Check sheet for the modelled part. Datum: model origin and axes. Units: mm. Face numbers are marked on the shaded views. A direction names the side the tool comes from. Round coordinates to 2 decimals unless told otherwise and drop trailing zeros. Order: outer loops, then holes, each group sorted by start corner. A loop starts at its lowest first (then second) coordinate and runs counter-clockwise, first axis right, second up. Notation, with made-up numbers: (89, 50.25) -> (99, 50.25) arc R21 ccw to (99, 89.25) -> close; hole circle Ø10 at (15.5, 84). An arc over 180 degrees is marked (long way). Answer in a Markdown table with one row per item. Add a question column.
1. Sectioned sample at B-B, the plane y = -103.5. Record the boundary of the cut face in (x, z).
2. Draft check along X on the marked faces 4, 5 and 6. Enter one of: +X half, -X half, draft (parallel to the pull), parting line (faces both ways), or undercut.
3. Material ranges on L1, parallel to Y at x = -21, z = -54; L2, parallel to X at y = -60.5, z = -39; L3, parallel to X at y = -79, z = -50, recorded low to high. Write a range as from..to.
4. Depth check by flat-ended pin: P1, Ø6, axis at y = -40.5, z = 13, coming from the +X side; P2, Ø8, axis at x = -46.5, z = -39, coming from the -Y side; P3, Ø8.5, axis at x = -23, y = -77, coming from the -Z side. Enter the tip coordinate at first touch or a pass-through.
5. Sectioned sample at D-D, the plane x = -25. Record the boundary of the cut face in (y, z), then the cut area to 3 significant figures.
6. Access from +Z, -Z, +X, -X, +Y, -Y to the whole of each face (thin tool, end or side, straight path). Record for the marked faces 1, 2 and 3.
7. Sectioned sample at A-A, the plane x = 4.5. Record the boundary of the cut face in (y, z), then the cut area to 3 significant figures.
8. Sectioned sample at C-C, the plane z = -14.5. Count the separate pieces of the cut face and the enclosed holes in it, then the cut area to 3 significant figures.
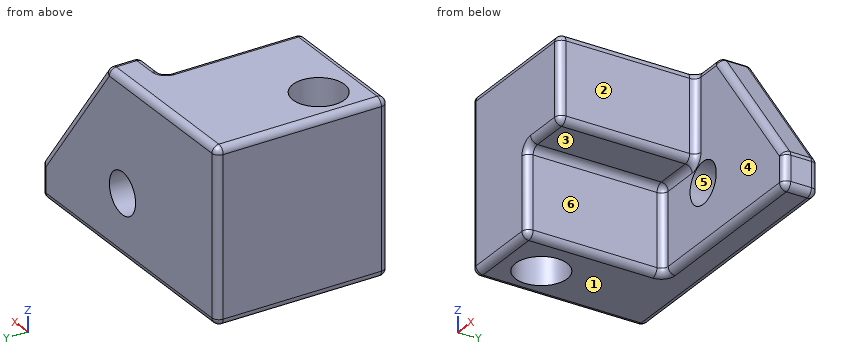
```python
from build123d import *

# Parameters (mm, degrees)
F0_W     = 203.2
F0_H     = 127
F1_DEPTH = 127
F3_DEPTH = 101.6
F4_SIZE2 = 101.6
F4_SIZE  = 76.2
F5_R     = 5.08
F6_R     = 15.24
F7_DEPTH = 25.4
F8_R     = 19.05
F9_DEPTH = 127


with BuildPart() as f1:
    # F0 (on Front) → F1 (new body)
    with BuildSketch(Plane.XZ):
        with Locations((-8.4275533497, -0.4033995528)):
            Rectangle(F0_W, F0_H)
    extrude(amount=F1_DEPTH)

    # F2 (on face) → F3 (cut)
    with BuildSketch(Plane.XZ.offset(127)):
        Polygon((-46.5275533497, -0.4033995528), (-46.5275533497, -63.9033995528), (93.1724466503, -63.9033995528), (93.1724466503, 63.0966004472), (-8.4275533497, 63.0966004472), (-8.4275533497, -0.4033995528), align=None)
    extrude(amount=-F3_DEPTH, mode=Mode.SUBTRACT)

    # F4
    f4_edges = [f1.edges().sort_by_distance(p)[0] for p in [
        (93.172447, -12.7, 63.0966),
    ]]
    f4_side = f1.faces().sort_by_distance((-42.29422, -55.033333, 63.0966))[0]
    chamfer(f4_edges, length=F4_SIZE, length2=F4_SIZE2, reference=f4_side)

    # F5
    f5_edges = [f1.edges().sort_by_distance(p)[0] for p in [
        (-46.527553, 0, 63.0966),
        (16.972447, -12.7, 63.0966),
        (-110.027553, -63.5, 63.0966),
        (4.272447, -25.4, 63.0966),
        (-59.227553, -127, 63.0966),
        (-8.427553, -76.2, 63.0966),
        (-8.427553, -127, 31.3466),
        (-27.477553, -127, -0.4034),
        (-46.527553, -127, -32.1534),
        (-78.277553, -127, -63.9034),
        (-110.027553, -127, -0.4034),
        (-8.427553, -76.2, -0.4034),
        (-8.427553, -25.4, 31.3466),
        (-46.527553, -76.2, -0.4034),
        (-46.527553, -76.2, -63.9034),
        (-46.527553, -25.4, -32.1534),
        (93.172447, -25.4, -51.2034),
        (55.072447, -25.4, 12.2966),
        (23.322447, -25.4, -63.9034),
        (-27.477553, -25.4, -0.4034),
        (55.072447, 0, 12.2966),
        (93.172447, -12.7, -38.5034),
        (93.172447, 0, -51.2034),
        (93.172447, -12.7, -63.9034),
        (-110.027553, -63.5, -63.9034),
        (-110.027553, 0, -0.4034),
        (-8.427553, 0, -63.9034),
    ]]
    fillet(f5_edges, radius=F5_R)

    # F6 (on face) → F7 (cut, through all)
    with BuildSketch(Plane.XZ.offset(25.4)):
        with Locations((-0.8075533497, -18.1833995528)):
            Circle(F6_R)
    extrude(amount=-F7_DEPTH, mode=Mode.SUBTRACT)

    # F8 (on face) → F9 (cut, through all)
    with BuildSketch(Plane.XY.offset(63.0966004472)):
        with Locations((-81.0180455446, -93.9986258745)):
            Circle(F8_R)
    extrude(amount=-F9_DEPTH, mode=Mode.SUBTRACT)


solid = f1.part
```
Answer key:
| question | item | result |
|---|---|---|
| 1 | outline | (-110.03, -58.82) arc R5.08 ccw to (-104.95, -63.9) -> (-97.53, -63.9) -> (-97.53, 63.1) -> (-104.95, 63.1) arc R5.08 ccw to (-110.03, 58.02) -> close; (-64.51, -63.9) -> (-51.61, -63.9) arc R5.08 ccw to (-46.53, -58.82) -> (-46.53, -5.48) arc R5.08 cw to (-41.45, -0.4) -> (-13.51, -0.4) arc R5.08 ccw to (-8.43, 4.68) -> (-8.43, 58.02) arc R5.08 ccw to (-13.51, 63.1) -> (-64.51, 63.1) -> close |
| 2 | face 4 | draft |
| 2 | face 5 | undercut |
| 2 | face 6 | +X half |
| 3 | L1 | y = -25.4..0 |
| 3 | L2 | x = -110.03..-46.53 |
| 3 | L3 | x = -110.03..-92.76, -69.27..-46.53 |
| 4 | P1 | stops at x = -8.43 |
| 4 | P2 | stops at y = -126.88 |
| 4 | P3 | stops at z = -0.4 |
| 5 | outline | (-127, 4.68) arc R5.08 ccw to (-121.92, -0.4) -> (-30.48, -0.4) arc R5.08 cw to (-25.4, -5.48) -> (-25.4, -58.82) arc R5.08 ccw to (-20.32, -63.9) -> (-5.08, -63.9) arc R5.08 ccw to (0, -58.82) -> (0, 58.02) arc R5.08 ccw to (-5.08, 63.1) -> (-121.92, 63.1) arc R5.08 ccw to (-127, 58.02) -> close |
| 5 | area | 9,660 mm² |
| 6 | face 1 | -Z, +X, -X, +Y, -Y |
| 6 | face 2 | +Z, -Z, +X, -Y |
| 6 | face 3 | -Z, +X, -Y |
| 7 | outline | (-25.4, -58.82) arc R5.08 ccw to (-20.32, -63.9) -> (-5.08, -63.9) arc R5.08 ccw to (0, -58.82) -> (0, -32.47) -> (-25.4, -32.47) -> close; (-25.4, -3.9) -> (0, -3.9) -> (0, 58.02) arc R5.08 ccw to (-5.08, 63.1) -> (-20.32, 63.1) arc R5.08 ccw to (-25.4, 58.02) -> close |
| 7 | area | 2,480 mm² |
| 8 | separate pieces | 2 |
| 8 | enclosed holes | 1 |
| 8 | area | 9,240 mm² |
